For this review, use the dimensioned drawing (mm, ordinates from the lowest corner) and the shaded views. A direction names the side the tool comes from. Give positions to 0.01 mm unless a question says otherwise; leave off trailing zeros. Loops run counter-clockwise (first coordinate to the right, second up) from the corner with the lowest first, then second, coordinate; pieces in that order, holes last. Notation, with made-up numbers: (43, 79) -> (62, 79) arc R23 cw to (62, 93) -> close; hole circle Ø2 at (2.5, 43.25). An arc over 180 degrees is marked (long way). Write each question's results on one line, items separated by ' | '. Start each with the question number.
Q1. We need section A-A (x = 28). Write out the cut boundary in (y, z).
Q2. Insertion check: pin 1 Ø6 at (y, z) = (17.5, 17) entering from +X; pin 2 Ø2 at (y, z) = (29, 21) entering from -X; pin 3 Ø20 at (x, y) = (23, 26.5) entering from +Z. Each pin has a flat end and moves straight along its axis. Give the tip position at first contact, or say it passes through.
Q3. We need section C-C (z = 23.5). Write out the cut boundary in (x, y).
Q4. Machinability: for the marked faces 1, 2 and 3, which of the approach directions +Z, -Z, +X, -X, +Y, -Y give a long, thin tool a straight path to every point of the face, cutting with its end or side? Answer none if there is none.
Q5. Mouldability with a two-part tool opening along X and no side actions: class the marked faces 4, 5, 6 and 7 as released by +X, released by -X, zero draft, split by the parting line, or undercut.
Q6. We need section B-B (y = 15). Give the number of separate pieces and of enclosed holes in the cut face, plus the area to 3 significant figures.
Q7. Wall thickness on L1, parallel to X at y = 20, z = 6; L2, parallel to Y at x = 100, z = 2.75; L3, parallel to Z at x = 60, y = 9: over which ranges is each line inside the solid? List them lowest first. Write a range as [from, to].
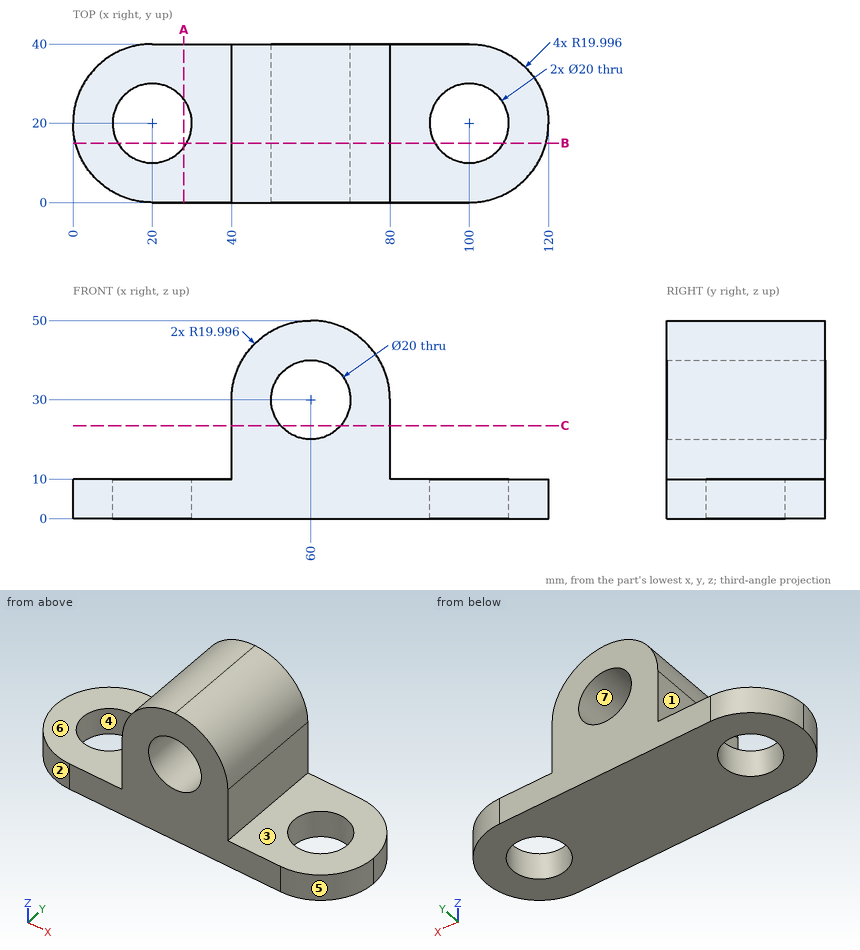
Output:
1) outline: (0, 0) -> (14, 0) -> (14, 10) -> (0, 10) -> close; (26, 0) -> (40, 0) -> (40, 10) -> (26, 10) -> close
2) pin 1: x = 80 | pin 2: x = 40 | pin 3: z = 10
3) outline: (40, 0) -> (52.4, 0) -> (52.4, 40) -> (40, 40) -> close; (67.6, 0) -> (80, 0) -> (80, 40) -> (67.6, 40) -> close
4) face 1: +Z, -X, +Y, -Y | face 2: +Z, -Z, -X, -Y | face 3: +Z, +X, +Y, -Y
5) face 4: undercut | face 5: released by +X | face 6: zero draft | face 7: undercut
6) separate pieces: 3 | enclosed holes: 1 | area: 1,960 mm2
7) L1: [0, 10], [30, 90], [110, 120] | L2: [0, 10], [30, 40] | L3: [0, 20], [40, 50]
